Can you work these out from the model? Positions are in its coordinate system, mm. A direction names the side the tool comes from. Coordinates: 2 decimals unless noted, no trailing zeros. Order: outer loops, then holes, each group sorted by start corner. A loop starts at its lowest first (then second) coordinate and runs counter-clockwise, first axis right, second up. Notation, with made-up numbers: (10.25, -10) -> (58.25, -10) arc R17 cw to (58.25, 6) -> close; hole circle Ø10 at (83, -3). An arc over 180 degrees is marked (long way). Answer as a JSON object with one key per item and string values. Group by question number.
(1) I need wall thicknesses on line 1 (X direction, y = 1, z = 0); line 2 (X direction, y = 14, z = -2); line 3 (Y direction, x = -5, z = 8). Which ranges of each line are inside material? Lowest first, please.
(2) For pin 1 (19 mm diameter, centred on x = -6, y = 18, fed in from +Z); pin 2 (3 mm diameter, centred on x = -3.5, z = 2.5, fed in from -Y); pin 3 (11 mm diameter, centred on x = -35, z = 0, fed in from +Y); pin 4 (5 mm diameter, centred on x = -6, y = 28.5, fed in from +Z), each with a flat end and sliding along its axis, tell me the tip position at first contact or that it passes through.
(3) I want a section at A-A, the plane x = 12.5. List the corners of the cut face in (y, z) for me, plus the area to 3 significant figures.
(4) If we mould it in two halves opening along Y, with no side actions, what happens to faces 4 (the cylindrical face through (-24.096, 25.18, 8.201)), 5 (the cylindrical face through (34.523, 1.479, -0.661)), 6 (the flat face through (0, 38, 0)), 7 (the cylindrical face through (26, 25, 10))? For each: pulls with the +Y half, pulls with the -Y half, needs draft (parallel to the pull), parting line crosses it, or undercut.
(5) I want a section at C-C, the plane z = -1.25. State how many separate pieces and enclosed holes the cut face has, plus the area to 3 significant figures.
(6) I want a section at B-B, the plane y = 4.5. List the corners of the cut face in (x, z) for me, plus the area to 3 significant figures.
(7) Which directions (+Z, -Z, +X, -X, +Y, -Y) give clear straight access to the entire face, cutting with the end or side of a thin tool? Please do faces 1 (the flat face through (-23, 29, 11.75)), 2 (the cylindrical face through (-25.54, 27.3, 10.23)), 3 (the flat face through (17.5, 1, 19)).
(8) I want a section at D-D, the plane z = 6. List the corners of the cut face in (x, y) for me, plus the area to 3 significant figures.
from build123d import *

# Parameters (mm, degrees)
SKICA1_W                 = 85
SKICA1_H                 = 17.5
SKICA1_R                 = 3.05
P_IDAT_VYSUNUT_M1_DEPTH  = 3
SKICA3_W                 = 65
SKICA3_H                 = 35
P_IDAT_VYSUNUT_M2_DEPTH  = 17.5
ZAOBLIT2_R               = 17
SKICA4_R                 = 6
SKICA4_R_2               = 4.1
P_IDAT_VYSUNUT_M3_DEPTH  = 3
SKICA4_2_R               = 4.1
ODEBRAT_VYSUNUT_M1_DEPTH = 4
SKICA5_W                 = 20
SKICA5_H                 = 15
ODEBRAT_VYSUNUT_M2_DEPTH = 60.636398282
SKICA7_R                 = 3.25
ODEBRAT_VYSUNUT_M4_DEPTH = 50
SKICA8_W                 = 35
SKICA8_H                 = 21
SKICA8_R                 = 3.05
P_IDAT_VYSUNUT_M4_DEPTH  = 3
ZAOBLIT1_R               = 4
EBRO4_REACH              = 66.306
SKICA12_WALL_W           = 153.460110402
SKICA12_WALL_H           = 10


with BuildPart() as part:
    # Skica1 → P_idat vysunut_m1 (new body)
    with BuildSketch(Plane(origin=(0, 0, 0), x_dir=(1, 0, 0), z_dir=(0, 1, 0))):
        Rectangle(SKICA1_W, SKICA1_H)
        with Locations(Location((-37.5, 0, 0), (0, 0, 270))):
            Circle(SKICA1_R, mode=Mode.SUBTRACT)
        with Locations(Location((37.5, 0, 0), (0, 0, 270))):
            Circle(SKICA1_R, mode=Mode.SUBTRACT)
    extrude(amount=P_IDAT_VYSUNUT_M1_DEPTH)

    # Skica3 → P_idat vysunut_m2 (add)
    with BuildSketch(Plane.XY.offset(8.75)):
        with Locations((0, 20.5)):
            Rectangle(SKICA3_W, SKICA3_H)
    extrude(amount=-P_IDAT_VYSUNUT_M2_DEPTH)

    # Zaoblit2
    zaoblit2_edges = [part.edges().sort_by_distance(p)[0] for p in [
        (32.5, 38, 0),
        (-32.5, 38, 0),
    ]]
    fillet(zaoblit2_edges, radius=ZAOBLIT2_R)

    # Skica4 → P_idat vysunut_m3 (add)
    with BuildSketch(Plane.XY.offset(8.75)):
        with Locations(Location((-20, 25, 0), (0, 0, 180))):
            Circle(SKICA4_R)
        with Locations((-20, 25)):
            Circle(SKICA4_R_2, mode=Mode.SUBTRACT)
        with Locations(Location((20, 25, 0), (0, 0, 180))):
            Circle(SKICA4_R)
        with Locations((20, 25)):
            Circle(SKICA4_R_2, mode=Mode.SUBTRACT)
    extrude(amount=P_IDAT_VYSUNUT_M3_DEPTH)

    # Skica4_2 → Odebrat vysunut_m1 (cut)
    with BuildSketch(Plane.XY.offset(8.75)):
        with Locations((20, 25)):
            Circle(SKICA4_2_R)
        with Locations((-20, 25)):
            Circle(SKICA4_2_R)
    extrude(amount=-ODEBRAT_VYSUNUT_M1_DEPTH, mode=Mode.SUBTRACT)

    # Skica5 → Odebrat vysunut_m2 (cut, through all)
    with BuildSketch(Plane.XY.offset(8.75)):
        with Locations((0, 19.5)):
            Rectangle(SKICA5_W, SKICA5_H)
    extrude(amount=-ODEBRAT_VYSUNUT_M2_DEPTH, mode=Mode.SUBTRACT)

    # Skica7 → Odebrat vysunut_m4 (cut)
    with BuildSketch(Plane(origin=(32.5, 0, 0), x_dir=(0, 0, -1), z_dir=(1, 0, 0))):
        with Locations(Location((1.25, 19.5, 0), (0, 0, 90))):
            Circle(SKICA7_R)
    extrude(amount=-ODEBRAT_VYSUNUT_M4_DEPTH, mode=Mode.SUBTRACT)

    # Skica8 → P_idat vysunut_m4 (add)
    with BuildSketch(Plane.XZ):
        with Locations((0, 19.25)):
            Rectangle(SKICA8_W, SKICA8_H)
        with Locations(Location((-12.5, 25, 0), (0, 0, 270))):
            Circle(SKICA8_R, mode=Mode.SUBTRACT)
        with Locations(Location((12.5, 25, 0), (0, 0, 90))):
            Circle(SKICA8_R, mode=Mode.SUBTRACT)
    extrude(amount=-P_IDAT_VYSUNUT_M4_DEPTH)

    # Zaoblit1
    zaoblit1_edges = [part.edges().sort_by_distance(p)[0] for p in [
        (17.5, 1.5, 8.75),
        (-17.5, 1.5, 8.75),
        (-17.5, 1.5, 29.75),
        (17.5, 1.5, 29.75),
        (42.5, 1.5, 8.75),
        (-42.5, 1.5, 8.75),
        (-42.5, 1.5, -8.75),
        (42.5, 1.5, -8.75),
    ]]
    fillet(zaoblit1_edges, radius=ZAOBLIT1_R)

    # Skica12 wall → ebro4 (add, up to next)
    with BuildSketch(Plane(origin=(0, 7.5, 19.25), x_dir=(0, 0.393919298579, -0.919145030018), z_dir=(0, 0.919145030018, 0.393919298579)), mode=Mode.PRIVATE) as ebro4_sk1:
        Rectangle(SKICA12_WALL_W, SKICA12_WALL_H)
    ebro4_tool1 = extrude(ebro4_sk1.sketch, amount=-EBRO4_REACH, mode=Mode.PRIVATE) - part.part
    add(ebro4_tool1.solids().sort_by_distance((0, 7.5, 19.25))[0])


solid = part.part
Computed values:
{
 "1": {"line 1": "x = -42.5 to -40.55, -34.45 to 34.45, 40.55 to 42.5", "line 2": "x = -32.5 to -10, 10 to 32.5", "line 3": "y = 0 to 12, 27 to 38"},
 "2": {"pin 1": "stops at z = 16.79", "pin 2": "stops at y = 0", "pin 3": "stops at y = 30.64", "pin 4": "stops at z = 8.75"},
 "3": {"outline": "(0, -8.75) -> (38, -8.75) -> (38, 8.75) -> (3, 8.75) -> (3, 21.95) -> (0, 21.95) -> close; (0, 28.05) -> (3, 28.05) -> (3, 29.75) -> (0, 29.75) -> close; hole circle Ø6.5 at (19.5, -1.25)", "area": "677 mm2"},
 "4": {"face 4": "undercut", "face 5": "needs draft", "face 6": "pulls with the +Y half", "face 7": "undercut"},
 "5": {"separate pieces": "3", "enclosed holes": "0", "area": "1,880 mm2"},
 "6": {"outline": "(-32.5, -8.75) -> (32.5, -8.75) -> (32.5, 8.75) -> (5, 8.75) -> (5, 26.25) -> (-5, 26.25) -> (-5, 8.75) -> (-32.5, 8.75) -> close", "area": "1,310 mm2"},
 "7": {"face 1": "+Z, +X, -X, +Y", "face 2": "+Z", "face 3": "+Z, +X, +Y, -Y"},
 "8": {"outline": "(-42.3, 0) -> (42.3, 0) -> (42.3, 3) -> (32.5, 3) -> (32.5, 21) arc R17 ccw to (15.5, 38) -> (-15.5, 38) arc R17 ccw to (-32.5, 21) -> (-32.5, 3) -> (-42.3, 3) -> close; hole circle Ø8.2 at (-20, 25); hole (-10, 12) -> (10, 12) -> (10, 27) -> (-10, 27) -> close; hole circle Ø8.2 at (20, 25)", "area": "2,000 mm2"}
}
